Part model, mm, in its own coordinate system. A direction names the side the tool comes from. Give positions to 0.01 mm unless a question says otherwise; leave off trailing zeros. Order: outer loops, then holes, each group sorted by start corner. A loop starts at its lowest first (then second) coordinate and runs counter-clockwise, first axis right, second up. Notation, with made-up numbers: M 27.25,60.5 L 84.25,60.5 A19 cw 84.25,83.5 Z; hole C 22.25,21.5 d6. An arc over 180 degrees is marked long. One line per question, with ' | ' between items.
```python
from build123d import *

# Parameters (mm, degrees)
F0_W     = 20
F0_H     = 13
F1_DEPTH = 5
F2_W     = 20
F2_H     = 2
F3_DEPTH = 20
F4_R     = 5
F7_DEPTH = 25
F5_R     = 1.5
F8_DEPTH = 25


with BuildPart() as f1:
    # F0 (on Top) → F1 (new body)
    with BuildSketch(Plane.XY):
        with Locations((10, 6.5)):
            Rectangle(F0_W, F0_H)
    extrude(amount=F1_DEPTH)

    # F2 (on face) → F3 (join)
    with BuildSketch(Plane.XY.offset(5)):
        with Locations((10, 12)):
            Rectangle(F2_W, F2_H)
    extrude(amount=F3_DEPTH)

    # F4
    f4_edges = [f1.edges().sort_by_distance(p)[0] for p in [
        (0, 12, 25),
        (20, 12, 25),
    ]]
    fillet(f4_edges, radius=F4_R)

    # F6 (on face) → F7 (cut)
    with BuildSketch(Plane(origin=(0, 0, 0), x_dir=(0, -1, 0), z_dir=(-1, 0, 0))):
        Polygon((-11, 25), (-12.5, 25), (-11, 15), align=None)
    extrude(amount=-F7_DEPTH, mode=Mode.SUBTRACT)

    # F5 (on face) → F8 (cut)
    with BuildSketch(Plane.XY.offset(5)):
        with Locations((10, 9.8)):
            Circle(F5_R)
    extrude(amount=-F8_DEPTH, mode=Mode.SUBTRACT)


solid = f1.part
```
1. Drop flat-ended pins along their axis: pin 1 (2 mm diameter, centred on x = 7.5, z = 15.5, fed in from -Y); pin 2 (4 mm diameter, centred on x = 12.5, z = 20.5, fed in from -Y) (3 decimals); pin 3 (5.5 mm diameter, centred on x = 11, y = 4, fed in from +Z). Give the stop position or say it passes through.
Worked out:
pin 1: stops at y = 11 | pin 2: stops at y = 11.525 | pin 3: stops at z = 5
2. Probe L1, parallel to Y at x = 10, z = 1.2; L2, parallel to X at y = 9.8, z = 2; L3, parallel to Y at x = 2, z = 8.25. List the from-to ranges inside material, lowest first. Write a range as from..to.
Worked out:
L1: y = 0..8.3, 11.3..13 | L2: x = 0..8.5, 11.5..20 | L3: y = 11..13
3. Slice it at B-B on y = 9.8. Give the cut face in (x, z), then the cut area to 3 significant figures.
Worked out:
outline: M 0,0 L 8.5,0 L 8.5,5 L 0,5 Z; M 11.5,0 L 20,0 L 20,5 L 11.5,5 Z | area: 85.0 mm2
4. Slice it at A-A on x = 10. Give the cut face in (y, z), then the cut area to 3 significant figures.
Worked out:
outline: M 0,0 L 8.3,0 L 8.3,5 L 0,5 Z; M 11,5 L 11.3,5 L 11.3,0 L 13,0 L 13,25 L 12.5,25 L 11,15 Z | area: 82.5 mm2
5. Slice it at C-C on z = 3. Give the cut face in (x, y).
Worked out:
outline: M 0,0 L 20,0 L 20,13 L 0,13 Z; hole C 10,9.8 d3
6. Tool access for faces 4 (the flat face through (10, 6, 5)), 5 (the flat face through (0, 7.9, 4.8)): list every direction of +Z, -Z, +X, -X, +Y, -Y with a clear straight run to the whole face (end or side of a thin tool).
Worked out:
face 4: +Z, +X, -X, -Y | face 5: +Z, -Z, -X, +Y, -Y
7. Slice it at D-D on x = 12.5. Give the cut face in (y, z), then the cut area to 3 significant figures.
Worked out:
outline: M 0,0 L 13,0 L 13,25 L 12.5,25 L 11,15 L 11,5 L 0,5 Z | area: 97.5 mm2
8. Mould opens along Y. For faces 1 (the flat face through (20, 7.9, 4.8)), 2 (the flat face through (10, 11, 10)), 3 (the cylindrical face through (8.8, 8.9, 2.5)) say: released by +Y, released by -Y, zero draft, split by the parting line, or undercut.
Worked out:
face 1: zero draft | face 2: released by -Y | face 3: undercut
